Study the drawing (mm; zero at the part's minimum x, y, z) and answer. Give positions to 0.01 mm unless a question says otherwise; leave off trailing zeros. Order: outer loops, then holes, each group sorted by start corner. A loop starts at its lowest first (then second) coordinate and runs counter-clockwise, first axis right, second up. Notation, with made-up numbers: (89, 83.5) - (103, 83.5) arc R13 ccw to (103, 103.5) - close; hole circle Ø3 at (46.5, -8). An arc over 180 degrees is marked (long way). Write each question's results on one line, items separated by ' | '. Start each with the question number.
Q1. Find section C-C on z = 1.05. Give the vertices of the cut face in (x, y) (1 decimal), and give its area (3 significant figures).
Q2. Flat-ended cylindrical pins translate along their axes: P1, Ø1.5, axis at x = 16.5, z = 1, coming from the -Y side; P2, Ø1.5, axis at x = 26.5, z = 0.5, coming from the +Y side. Find the tip coordinate at first contact, or state that the pin passes through.
Q3. Find section D-D on y = 27.5. Give the vertices of the cut face in (x, z) (1 decimal).
Q4. Find section B-B on y = 38.1. Give the vertices of the cut face in (x, z), and give its area (3 significant figures).
Q5. Find the intervals of material crossed by line 1 along Y through (x, z) = (38.1, 2.2); line 2 along Y through (x, z) = (43, 0.85); line 3 along X through (y, z) = (48.5, 1.05), in increasing order. Write a range as from..to.
Q6. Find section A-A on x = 38.1. Give the vertices of the cut face in (y, z).
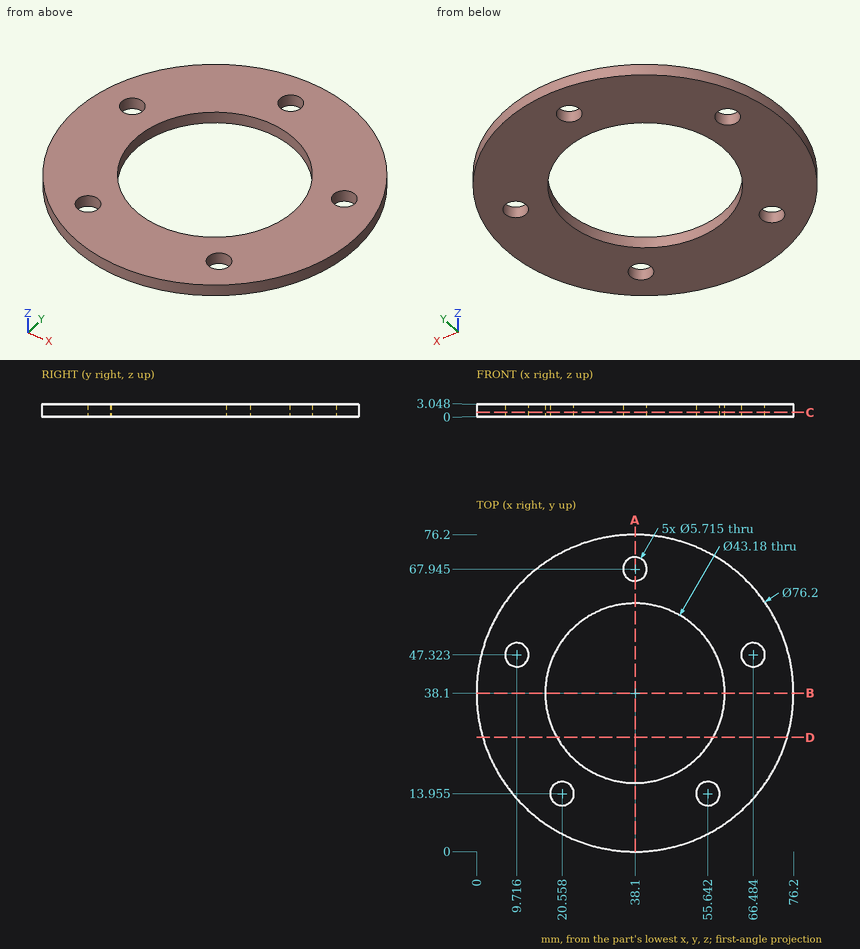
Working result:
1) outline: circle Ø76.2 at (38.1, 38.1); hole circle Ø5.7 at (9.7, 47.3); hole circle Ø43.2 at (38.1, 38.1); hole circle Ø5.7 at (20.6, 14); hole circle Ø5.7 at (38.1, 67.9); hole circle Ø5.7 at (55.6, 14); hole circle Ø5.7 at (66.5, 47.3) | area: 2,970 mm²
2) P1: y = 6.21 | P2: y = 74.62
3) outline: (1.5, 0) - (19.3, 0) - (19.3, 3) - (1.5, 3) - close; (56.9, 0) - (74.7, 0) - (74.7, 3) - (56.9, 3) - close
4) outline: (0, 0) - (16.51, 0) - (16.51, 3.05) - (0, 3.05) - close; (59.69, 0) - (76.2, 0) - (76.2, 3.05) - (59.69, 3.05) - close | area: 101 mm²
5) line 1: 0..16.51, 59.69..65.09, 70.8..76.2 | line 2: 0.32..17.07, 59.13..75.88 | line 3: 1.45..7.11, 12.32..19.18, 57.02..63.88, 69.09..74.75
6) outline: (0, 0) - (16.51, 0) - (16.51, 3.05) - (0, 3.05) - close; (59.69, 0) - (65.09, 0) - (65.09, 3.05) - (59.69, 3.05) - close; (70.8, 0) - (76.2, 0) - (76.2, 3.05) - (70.8, 3.05) - close
